```python
from build123d import *

# Parameters (mm, degrees)
PAD039_DEPTH    = 50
POCKET035_DEPTH = 132.001
SKETCH113_R     = 2.3
POCKET036_DEPTH = 5.5
SKETCH114_R     = 1.7
HOLE022_DEPTH   = 25
SKETCH115_R     = 2.5
POCKET037_DEPTH = 17.001


with BuildPart() as part:
    # Sketch111 → Pad039 (new body)
    with BuildSketch(Plane.YZ):
        Polygon((106, 235), (132, 235), (132, 218), (126, 218), (126, 228), (106, 228), align=None)
    extrude(amount=PAD039_DEPTH)

    # Sketch112 → Pocket035 (cut, through all)
    with BuildSketch(Plane.XZ):
        Polygon((20, 218), (0, 218), (0, 228), (6, 228), align=None)
        Polygon((30, 218), (50, 218), (50, 228), (44, 228), align=None)
    extrude(amount=-POCKET035_DEPTH, mode=Mode.SUBTRACT)

    # Sketch113 (on Face1 of Pocket035) → Pocket036 (cut)
    with BuildSketch(Plane(origin=(0, 0, 235), x_dir=(0, -1, 0), z_dir=(0, 0, 1))):
        with Locations((-119, 42.5)):
            Circle(SKETCH113_R)
        with Locations((-119, 5.5)):
            Circle(SKETCH113_R)
    extrude(amount=-POCKET036_DEPTH, mode=Mode.SUBTRACT)

    # Sketch114 (on Face18 of Pocket036) → Hole022 (cut)
    with BuildSketch(Plane(origin=(0, 126, 0), x_dir=(0, 0, -1), z_dir=(0, -1, 0))):
        with Locations((-224.5, 32.5)):
            Circle(SKETCH114_R)
        with Locations((-224.5, 17.5)):
            Circle(SKETCH114_R)
    extrude(amount=-HOLE022_DEPTH, mode=Mode.SUBTRACT)

    # Sketch115 (on Face1 of Hole022) → Pocket037 (cut, through all)
    with BuildSketch(Plane(origin=(0, 0, 235), x_dir=(0, -1, 0), z_dir=(0, 0, 1))):
        with Locations((-119, 25)):
            Circle(SKETCH115_R)
    extrude(amount=-POCKET037_DEPTH, mode=Mode.SUBTRACT)


with BuildPart() as part_1:
    # Body016 placement: moved
    add(part.part.moved(Location((-25, 0, 0))))


solid = part_1.part
```
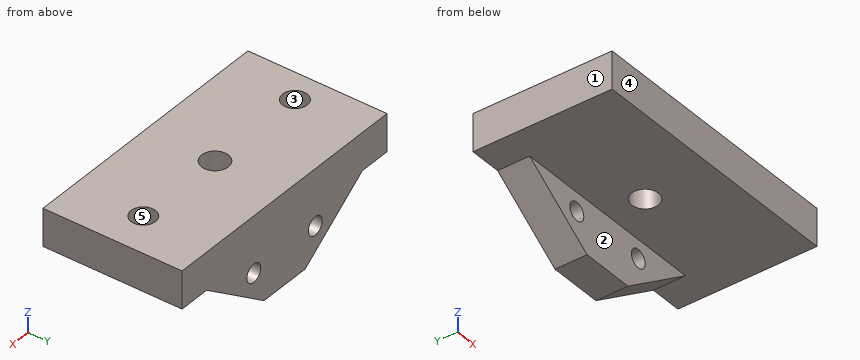
Geometry check sheet. Reference: the model listing, model coordinates, mm. Face numbers are marked on the shaded views. A direction names the side the tool comes from. Coordinates: 2 decimals unless noted, no trailing zeros. Order: outer loops, then holes, each group sorted by start corner. A loop starts at its lowest first (then second) coordinate and runs counter-clockwise, first axis right, second up. Notation, with made-up numbers: M 11.25,49 L 37.25,49 A18 cw 37.25,73 Z; hole C 77,29.25 d5. An arc over 180 degrees is marked long. One line per question, with ' | ' between items. Start each with the question number.
Item 1: Cross-section at B-B on z = 228.5. Enter the section's corners in (x, y).
Item 2: Gauge pin test, flat ends, axial feed: pin 1 (3 mm diameter, centred on x = -11, y = 110, fed in from -Z); pin 2 (3 mm diameter, centred on x = 2, z = 225, fed in from -Y); pin 3 (3.5 mm diameter, centred on x = -19.5, y = 119, fed in from +Z). Record the tip position at first contact, or that the pin passes through.
Item 3: Material ranges on L1, parallel to X at y = 119, z = 231.3; L2, parallel to X at y = 119, z = 228.5; L3, parallel to X at y = 128.1, z = 224.5, recorded low to high. Write a range as [from, to].
Item 4: Cross-section at C-C on x = 0. Enter the section's corners in (y, z), then the cut area to 3 significant figures.
Item 5: Cross-section at D-D on z = 224.5. Enter the section's corners in (x, y), then the cut area to 3 significant figures.
Item 6: Cross-section at A-A on y = 119. Enter the section's corners in (x, z).
Item 7: Set-up check for the marked faces 4 and 5: record each of +Z, -Z, +X, -X, +Y, -Y from which the full face is reachable in a straight line by a thin tool's end or side.
Item 8: Draft check along X on the marked faces 1, 2 and 3. Enter one of: pulls with the +X half, pulls with the -X half, needs draft (parallel to the pull), parting line crosses it, or undercut.
Findings:
1) outline: M -25,106 L 25,106 L 25,132 L -25,132 Z; hole C 0,119 d5
2) pin 1: stops at z = 228 | pin 2: stops at y = 126 | pin 3: stops at z = 229.5
3) L1: x = [-25, -21.8], [-17.2, -2.5], [2.5, 15.2], [19.8, 25] | L2: x = [-25, -2.5], [2.5, 25] | L3: x = [-14.1, -9.2], [-5.8, 5.8], [9.2, 14.1]
4) outline: M 106,228 L 116.5,228 L 116.5,235 L 106,235 Z; M 121.5,228 L 126,228 L 126,218 L 132,218 L 132,235 L 121.5,235 Z | area: 207 mm²
5) outline: M -14.1,126 L -9.2,126 L -9.2,132 L -14.1,132 Z; M -5.8,126 L 5.8,126 L 5.8,132 L -5.8,132 Z; M 9.2,126 L 14.1,126 L 14.1,132 L 9.2,132 Z | area: 128 mm²
6) outline: M -25,228 L -2.5,228 L -2.5,235 L -17.2,235 L -17.2,229.5 L -21.8,229.5 L -21.8,235 L -25,235 Z; M 2.5,228 L 25,228 L 25,235 L 19.8,235 L 19.8,229.5 L 15.2,229.5 L 15.2,235 L 2.5,235 Z
7) face 4: +Z, -Z, +X, -X, -Y | face 5: +Z
8) face 1: pulls with the -X half | face 2: needs draft | face 3: undercut
